Model file for the job. Use its own axes, mm. Face numbers are marked on the shaded views. Give positions to 0.01 mm unless a question says otherwise; leave off trailing zeros. Loops run counter-clockwise (first coordinate to the right, second up) from the corner with the lowest first, then second, coordinate; pieces in that order, holes last. Notation, with made-up numbers: M -3,48 L 7,48 A31 ccw 7,83 Z; hole C 24.25,75 d5. An arc over 180 degrees is marked long. Answer in a Markdown table with one row per item.
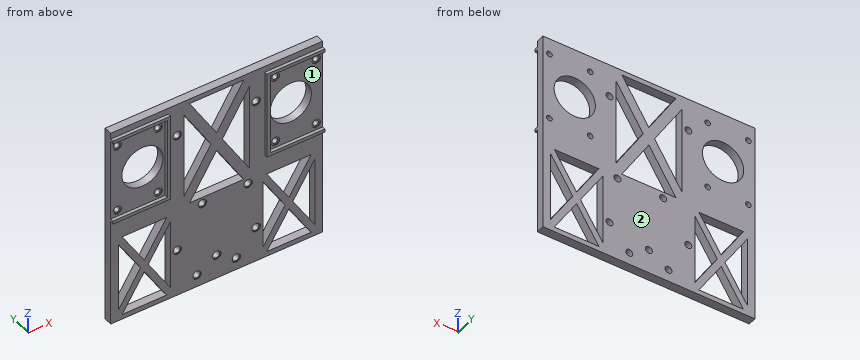
```python
from build123d import *

# Parameters (mm, degrees)
SKETCH1_W           = 130
SKETCH1_H           = 125
BOSS_EXTRUDE1_DEPTH = 5
SKETCH2_R           = 1.75
SKETCH2_R_2         = 12.65
CUT_EXTRUDE1_DEPTH  = 10
SKETCH3_R           = 2.15
CUT_EXTRUDE2_DEPTH  = 10
SKETCH4_R           = 2.15
CUT_EXTRUDE3_DEPTH  = 10
BOSS_EXTRUDE2_DEPTH = 2
SKETCH6_R           = 2.65
CUT_EXTRUDE4_DEPTH  = 0.5
CUT_EXTRUDE5_DEPTH  = 91.311959341
CUT_EXTRUDE6_DEPTH  = 91.311959341


with BuildPart() as part:
    # Sketch1 → Boss-Extrude1 (new body)
    with BuildSketch(Plane(origin=(0, 0, 0), x_dir=(1, 0, 0), z_dir=(0, 1, 0))):
        Rectangle(SKETCH1_W, SKETCH1_H)
    extrude(amount=BOSS_EXTRUDE1_DEPTH)

    # Sketch2 → Cut-Extrude1 (cut)
    with BuildSketch(Plane(origin=(0, 5, 0), x_dir=(1, 0, 0), z_dir=(0, 1, 0))):
        with Locations(Location((-61, -52.5, 0), (0, 0, 270))):
            Circle(SKETCH2_R)
        with Locations(Location((-36, -52.5, 0), (0, 0, 270))):
            Circle(SKETCH2_R)
        with Locations(Location((-36, -10.5, 0), (0, 0, 270))):
            Circle(SKETCH2_R)
        with Locations(Location((-61, -10.5, 0), (0, 0, 270))):
            Circle(SKETCH2_R)
        with Locations(Location((-45.5, -31.5, 0), (0, 0, 270))):
            Circle(SKETCH2_R_2)
    cut_extrude1 = extrude(amount=-CUT_EXTRUDE1_DEPTH, mode=Mode.SUBTRACT)

    # Mirror3: Cut-Extrude1 across plane
    add(cut_extrude1.mirror(Plane.ZY), mode=Mode.SUBTRACT)

    # Sketch3 → Cut-Extrude2 (cut)
    with BuildSketch(Plane(origin=(0, 5, 0), x_dir=(1, 0, 0), z_dir=(0, 1, 0))):
        with Locations(Location((-24.17, -42.03, 0), (0, 0, 270))):
            Circle(SKETCH3_R)
        with Locations(Location((24.17, -42.03, 0), (0, 0, 270))):
            Circle(SKETCH3_R)
        with Locations(Location((-8.73, 9.6, 0), (0, 0, 270))):
            Circle(SKETCH3_R)
        with Locations(Location((19.29, 9.6, 0), (0, 0, 270))):
            Circle(SKETCH3_R)
        with Locations(Location((-24.17, 33.11, 0), (0, 0, 270))):
            Circle(SKETCH3_R)
        with Locations(Location((24.17, 40.6, 0), (0, 0, 270))):
            Circle(SKETCH3_R)
    extrude(amount=-CUT_EXTRUDE2_DEPTH, mode=Mode.SUBTRACT)

    # Sketch4 → Cut-Extrude3 (cut)
    with BuildSketch(Plane(origin=(0, 5, 0), x_dir=(1, 0, 0), z_dir=(0, 1, 0))):
        with Locations(Location((0, 47.5, 0), (0, 0, 270))):
            Circle(SKETCH4_R)
        with Locations(Location((12.049810205, 55, 0), (0, 0, 270))):
            Circle(SKETCH4_R)
        with Locations(Location((-12.049810205, 55, 0), (0, 0, 270))):
            Circle(SKETCH4_R)
    extrude(amount=-CUT_EXTRUDE3_DEPTH, mode=Mode.SUBTRACT)

    # Sketch5 → Boss-Extrude2 (add)
    with BuildSketch(Plane.XZ):
        Polygon((-65, 58.7), (-65, 56.7), (-31.6, 56.7), (-31.6, 6.3), (-65, 6.3), (-65, 4.3), (-29.6, 4.3), (-29.6, 58.7), align=None)
    boss_extrude2 = extrude(amount=BOSS_EXTRUDE2_DEPTH)

    # Mirror5: Boss-Extrude2 across plane
    add(boss_extrude2.mirror(Plane.ZY))

    # Sketch6 → Cut-Extrude4 (cut)
    with BuildSketch(Plane.XZ):
        with Locations(Location((-12.049810205, -55, 0), (0, 0, 270))):
            Circle(SKETCH6_R)
        with Locations(Location((12.049810205, -55, 0), (0, 0, 270))):
            Circle(SKETCH6_R)
        with Locations(Location((0, -47.5, 0), (0, 0, 270))):
            Circle(SKETCH6_R)
        with Locations(Location((24.17, -40.6, 0), (0, 0, 270))):
            Circle(SKETCH6_R)
        with Locations(Location((-24.17, -33.11, 0), (0, 0, 270))):
            Circle(SKETCH6_R)
        with Locations(Location((-8.73, -9.6, 0), (0, 0, 270))):
            Circle(SKETCH6_R)
        with Locations(Location((19.29, -9.6, 0), (0, 0, 270))):
            Circle(SKETCH6_R)
        with Locations(Location((-61, 10.5, 0), (0, 0, 270))):
            Circle(SKETCH6_R)
        with Locations(Location((-61, 52.5, 0), (0, 0, 270))):
            Circle(SKETCH6_R)
        with Locations(Location((-36, 52.5, 0), (0, 0, 270))):
            Circle(SKETCH6_R)
        with Locations(Location((-36, 10.5, 0), (0, 0, 270))):
            Circle(SKETCH6_R)
        with Locations(Location((-24.17, 42.03, 0), (0, 0, 270))):
            Circle(SKETCH6_R)
        with Locations(Location((24.17, 42.03, 0), (0, 0, 270))):
            Circle(SKETCH6_R)
        with Locations(Location((36, 52.5, 0), (0, 0, 270))):
            Circle(SKETCH6_R)
        with Locations(Location((36, 10.5, 0), (0, 0, 270))):
            Circle(SKETCH6_R)
        with Locations(Location((61, 10.5, 0), (0, 0, 270))):
            Circle(SKETCH6_R)
        with Locations(Location((61, 52.5, 0), (0, 0, 270))):
            Circle(SKETCH6_R)
    extrude(amount=-CUT_EXTRUDE4_DEPTH, mode=Mode.SUBTRACT)

    # Sketch7 → Cut-Extrude5 (cut, through all)
    with BuildSketch(Plane.XZ):
        Polygon((-3.470107527, 26.95), (-20.17, 53.9), (-20.17, 0), align=None)
        Polygon((16.629937096, 59.5), (-16.629937096, 59.5), (0, 32.662892788), align=None)
        Polygon((20.17, 0), (20.17, 53.9), (3.470107527, 26.95), align=None)
        Polygon((0, 21.237107212), (-16.629937096, -5.6), (16.629937096, -5.6), align=None)
    extrude(amount=-CUT_EXTRUDE5_DEPTH, mode=Mode.SUBTRACT)

    # Sketch8 → Cut-Extrude6 (cut, through all)
    with BuildSketch(Plane.XZ):
        Polygon((-46.699325365, -34.05), (-60.372350745, -12.351497003), (-60.372350745, -55.748502997), align=None)
        Polygon((-30.662343644, -8.6), (-58.008394405, -8.6), (-44.335369025, -30.298502997), align=None)
        Polygon((-28.298387304, -55.748502997), (-28.298387304, -12.351497003), (-41.971412684, -34.05), align=None)
        Polygon((-44.335369025, -37.801497003), (-58.008394405, -59.5), (-30.662343644, -59.5), align=None)
        Polygon((41.971412684, -34.05), (28.298387304, -12.351497003), (28.298387304, -55.748502997), align=None)
        Polygon((44.335369025, -30.298502997), (58.008394405, -8.6), (30.662343644, -8.6), align=None)
        Polygon((60.372350745, -12.351497003), (46.699325365, -34.05), (60.372350745, -55.748502997), align=None)
        Polygon((30.662343644, -59.5), (58.008394405, -59.5), (44.335369025, -37.801497003), align=None)
    extrude(amount=-CUT_EXTRUDE6_DEPTH, mode=Mode.SUBTRACT)


solid = part.part
```
(1) Wall check: L1, parallel to X at y = 4, z = 29; L2, parallel to X at y = 2.25, z = 20.5; L3, parallel to Z at x = -53.5, y = 2. Give the ranges that are in metal, low to high.
Established:
| item | result |
|---|---|
| L1 | x = -65 to -57.9, -33.1 to -20.17, -4.74 to 4.74, 20.17 to 33.1, 57.9 to 65 |
| L2 | x = -65 to -51.75, -39.25 to -20.17, -7.47 to -0.46, 0.46 to 7.47, 20.17 to 39.25, 51.75 to 65 |
| L3 | z = -62.5 to -59.5, -52.35 to -44.84, -23.26 to -15.75, -8.6 to 21.7, 41.3 to 62.5 |
(2) Saw through at A-A, the plane x = 54. Give the cut face in (y, z).
Established:
| item | result |
|---|---|
| outline | M -2,4.3 L 0,4.3 L 0,-8.6 L 5,-8.6 L 5,22.13 L 0,22.13 L 0,6.3 L -2,6.3 Z; M -2,56.7 L 0,56.7 L 0,40.87 L 5,40.87 L 5,62.5 L 0,62.5 L 0,58.7 L -2,58.7 Z; M 0,-62.5 L 5,-62.5 L 5,-59.5 L 0,-59.5 Z; M 0,-53.14 L 5,-53.14 L 5,-45.64 L 0,-45.64 Z; M 0,-22.46 L 5,-22.46 L 5,-14.96 L 0,-14.96 Z |
(3) Saw through at B-B, the plane z = 30.5. Give the cut face in (x, y), and give its area (3 significant figures).
Established:
| item | result |
|---|---|
| outline | M -65,0 L -58.11,0 L -58.11,5 L -65,5 Z; M -32.89,0 L -31.6,0 L -31.6,-2 L -29.6,-2 L -29.6,0 L -20.17,0 L -20.17,5 L -32.89,5 Z; M -5.67,0 L 5.67,0 L 5.67,5 L -5.67,5 Z; M 20.17,0 L 29.6,0 L 29.6,-2 L 31.6,-2 L 31.6,0 L 32.89,0 L 32.89,5 L 20.17,5 Z; M 58.11,0 L 65,0 L 65,5 L 58.11,5 Z |
| area | 261 mm2 |
(4) Flat gauge pins, fed straight in: P1, Ø4, axis at x = -36, z = 52.5, coming from the -Y side; P2, Ø1.6, axis at x = -41.5, y = -1, coming from the +Z side; P3, Ø4, axis at x = 20, z = 41, coming from the -Y side. Where does each tip first touch, or does it go through?
Established:
| item | result |
|---|---|
| P1 | stops at y = 0.5 |
| P2 | stops at z = 58.7 |
| P3 | stops at y = 0 |
(5) Mould opens along Z. For the marked faces 1 and 2 say: pulls with the +Z half, pulls with the -Z half, needs draft (parallel to the pull), parting line crosses it, or undercut.
Established:
| item | result |
|---|---|
| face 1 | undercut |
| face 2 | needs draft |
(6) Saw through at C-C, the plane z = 10.5. Count the separate pieces of the cut face and the enclosed holes in it, and give its area (3 significant figures).
Established:
| item | result |
|---|---|
| separate pieces | 8 |
| enclosed holes | 0 |
| area | 453 mm2 |
